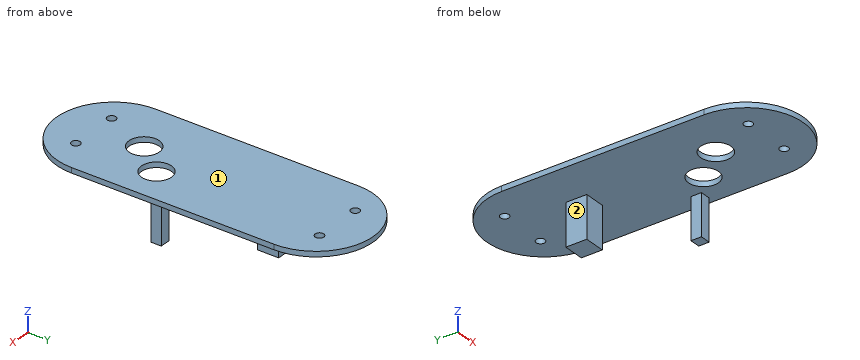
```python
from build123d import *

# Parameters (mm, degrees)
BOX026_W          = 4
BOX026_H          = 4
BOX026_DEPTH      = 15.8
BOX032_W          = 8
BOX032_H          = 8
BOX032_DEPTH      = 16
CYLINDER007_R     = 1.65
CYLINDER007_DEPTH = 6
SKETCH002_R       = 5.774373
SKETCH002_R_2     = 5.727235
EXTRUDE002_DEPTH  = 5
EXTRUDE004_DEPTH  = 2


with BuildPart() as spacer002:
    # Box026 → Box026 (new body)
    with BuildSketch(Plane(origin=(35, -32, 8.2), x_dir=(1, 0, 0), z_dir=(0, 0, 1))):
        with Locations((2, 2)):
            Rectangle(BOX026_W, BOX026_H)
    extrude(amount=BOX026_DEPTH)


with BuildPart() as spacer003:
    # Box032 → Box032 (new body)
    with BuildSketch(Plane(origin=(15, -3, 8), x_dir=(1, 0, 0), z_dir=(0, 0, 1))):
        with Locations((4, 4)):
            Rectangle(BOX032_W, BOX032_H)
    extrude(amount=BOX032_DEPTH)


with BuildPart() as hole006:
    # Cylinder007 → Cylinder007 (new body)
    with BuildSketch(Plane(origin=(10.5, 25, 23), x_dir=(1, 0, 0), z_dir=(0, 0, 1))):
        Circle(CYLINDER007_R)
    extrude(amount=CYLINDER007_DEPTH)


with BuildPart() as hole007:
    # Clone014 base: copy of hole006
    add(hole006.part)


with BuildPart() as hole007_1:
    # Clone014 placement: moved
    add(hole007.part.moved(Location((18.5, 0, 0))))


with BuildPart() as hole008:
    # Clone015 base: copy of hole007
    add(hole007_1.part)


with BuildPart() as hole008_1:
    # Clone015 placement: moved
    add(hole008.part.moved(Location((-18.5, -93, 0))))


with BuildPart() as hole009:
    # Clone016 base: copy of hole008
    add(hole008_1.part)


with BuildPart() as hole009_1:
    # Clone016 placement: moved
    add(hole009.part.moved(Location((18.5, 0, 0))))


with BuildPart() as knobholes001:
    # Sketch002 → Extrude002 (new body)
    with BuildSketch(Plane(origin=(11, -50, 24), x_dir=(1, 0, 0), z_dir=(0, 0, 1))):
        with Locations((7.047384, 0)):
            Circle(SKETCH002_R)
        with Locations((16.925785, 11.999866)):
            Circle(SKETCH002_R_2)
    extrude(amount=EXTRUDE002_DEPTH)


with BuildPart() as fusion005:
    # Fusion005 base: copy of hole006
    add(hole006.part)

    # Fusion005: union hole007, hole008, hole009, knobHoles001
    add(hole007_1.part)
    add(hole008_1.part)
    add(hole009_1.part)
    add(knobholes001.part)


with BuildPart() as lid003:
    # Clone2D → Extrude004 (new body)
    with BuildSketch(Plane(origin=(0, -60, 24), x_dir=(1, 0, 0), z_dir=(0, 0, 1))):
        with BuildLine():
            ThreePointArc((41.5, 76.908478), (19.75, 98.658478), (-2, 76.908478))
            Line((-2, 76.908478), (-2, -0.333569))
            ThreePointArc((-2, -0.333569), (19.75, -22.083569), (41.5, -0.333569))
            Line((41.5, -0.333569), (41.5, 76.908478))
        make_face()
    extrude(amount=EXTRUDE004_DEPTH)

    # Cut004: cut Fusion005
    add(fusion005.part, mode=Mode.SUBTRACT)

    # Fusion006: union spacer002, spacer003
    add(spacer002.part)
    add(spacer003.part)


solid = lid003.part
```
Source: CAD feature listing. Evaluate the final solid. Frame: model axes, mm. Face numbers are marked on the shaded views. A direction names the side the tool comes from. Round coordinates to 2 decimals unless told otherwise and drop trailing zeros. Loops run counter-clockwise (first coordinate to the right, second up) from the corner with the lowest first, then second, coordinate; pieces in that order, holes last.
(1) Material intervals for probe 1 along Y at (x, z) = (29, 24.5); probe 2 along Y at (x, z) = (10.5, 25.5); probe 3 along X at (y, z) = (-68, 24.65), sorted ascending.
From the geometry:
probe 1: y = -80.02 to -69.65, -66.35 to -43.63, -32.37 to 23.35, 26.65 to 36.59
probe 2: y = -80.02 to -69.65, -66.35 to 23.35, 26.65 to 36.59
probe 3: x = -0.6 to 8.85, 12.15 to 27.35, 30.65 to 40.1
(2) Section query A-A (y = -50). Output: boundary loops of the cut face in (x, z), and give its area (3 significant figures).
From the geometry:
outline: (-2, 24) - (12.27, 24) - (12.27, 26) - (-2, 26) - close; (23.82, 24) - (41.5, 24) - (41.5, 26) - (23.82, 26) - close
area: 63.9 mm2
(3) Contact query for flat-ended pins moving along their axis: pin 1 Ø6 at (y, z) = (-59.5, 19) entering from +X; pin 2 Ø5 at (y, z) = (2.5, 12.5) entering from -X; pin 3 Ø1.5 at (y, z) = (5.5, 14) entering from +X; pin 4 Ø1.2 at (x, y) = (36, -30.5) entering from -Z. Output: stop coordinate, or through.
From the geometry:
pin 1: passes through
pin 2: stops at x = 15
pin 3: stops at x = 23
pin 4: stops at z = 8.2
(4) Section query B-B (z = 14). Output: boundary loops of the cut face in (x, y).
From the geometry:
outline: (15, -3) - (23, -3) - (23, 5) - (15, 5) - close; (35, -32) - (39, -32) - (39, -28) - (35, -28) - close
(5) Section query D-D (x = 19). Output: boundary loops of the cut face in (y, z).
From the geometry:
outline: (-82.07, 24) - (-55.7, 24) - (-55.7, 26) - (-82.07, 26) - close; (-44.3, 24) - (-3, 24) - (-3, 8) - (5, 8) - (5, 24) - (38.65, 24) - (38.65, 26) - (-44.3, 26) - close
(6) Access query for the marked faces 1 and 2. Directions: +Z, -Z, +X, -X, +Y, -Y. A direction counts if a zero-diameter tool reaches every point of the face in a straight line with its end or side. Return the directions, or none.
From the geometry:
face 1: +Z, +X, -X, +Y, -Y
face 2: -Z, -X, +Y, -Y
(7) Section query C-C (x = 29). Output: boundary loops of the cut face in (y, z).
From the geometry:
outline: (-80.02, 24) - (-69.65, 24) - (-69.65, 26) - (-80.02, 26) - close; (-66.35, 24) - (-43.63, 24) - (-43.63, 26) - (-66.35, 26) - close; (-32.37, 24) - (23.35, 24) - (23.35, 26) - (-32.37, 26) - close; (26.65, 24) - (36.59, 24) - (36.59, 26) - (26.65, 26) - close
